Design review of the part built by this model. Coordinates are the model's own, in mm. A direction names the side the tool comes from. Coordinates: 2 decimals unless noted, no trailing zeros. Write each loop counter-clockwise with the first axis right and the second up, starting at its lowest first coordinate (ties: lowest second). Pieces come first, ordered by that corner, then holes. Notation, with made-up numbers: (-11, 43.5) - (10, 43.5) arc R33 ccw to (10, 76.5) - close; hole circle Ø3 at (61, 29.25). An arc over 180 degrees is marked (long way). Answer as a JSON object with one key per item and string values.
```python
from build123d import *

# Parameters (mm, degrees)
BOSS_EXTRUDE1_DEPTH         = 39.9
CUT_EXTRUDE1_DEPTH          = 1
CUT_EXTRUDE1_DEPTH_BACK     = 40.5
CUT_EXTRUDE2_DEPTH          = 1
CUT_EXTRUDE2_DEPTH_BACK     = 40.5
M4_TAPPED_HOLE1_D           = 3.3
M4_TAPPED_HOLE1_DEPTH       = 10.1
M4_TAPPED_HOLE1_CSINK_D     = 4.05
M4_TAPPED_HOLE1_CSINK_ANGLE = 90
M4_TAPPED_HOLE1_TIP         = 0.991420021
SKETCH6_W                   = 24.75
SKETCH6_H                   = 6.7
CUT_EXTRUDE3_DEPTH          = 2


with BuildPart() as part:
    # Sketch1 → Boss-Extrude1 (new body)
    with BuildSketch(Plane.XY):
        with BuildLine():
            Line((24.75, 0), (24.75, 14.75))
            Line((24.75, 14.75), (39.5, 14.75))
            Line((39.5, 14.75), (39.5, 39.5))
            Line((39.5, 39.5), (23.5, 39.5))
            Line((23.5, 39.5), (23.5, 20.25))
            ThreePointArc((23.5, 20.25), (22.181980515, 17.068019485), (19, 15.75))
            Line((19, 15.75), (0, 15.75))
            Line((0, 15.75), (0, 0))
            Line((0, 0), (24.75, 0))
        make_face()
    extrude(amount=BOSS_EXTRUDE1_DEPTH)

    # Sketch2 → Cut-Extrude1 (cut, two sides)
    with BuildSketch(Plane.XZ) as cut_extrude1_sk:
        with BuildLine():
            Line((10.3, 39.9), (12.3, 39.9))
            Line((12.3, 39.9), (12.3, 22.422616289))
            ThreePointArc((12.3, 22.422616289), (17.8, 16), (12.3, 9.577383711))
            Line((12.3, 9.577383711), (12.3, 2.9))
            Line((12.3, 2.9), (10.3, 2.9))
            Line((10.3, 2.9), (10.3, 9.577383711))
            ThreePointArc((10.3, 9.577383711), (4.8, 16), (10.3, 22.422616289))
            Line((10.3, 22.422616289), (10.3, 39.9))
        make_face()
    extrude(amount=CUT_EXTRUDE1_DEPTH, mode=Mode.SUBTRACT)
    extrude(cut_extrude1_sk.sketch, amount=-CUT_EXTRUDE1_DEPTH_BACK, mode=Mode.SUBTRACT)

    # Sketch3 → Cut-Extrude2 (cut, two sides)
    with BuildSketch(Plane(origin=(39.5, 0, 0), x_dir=(0, 0, -1), z_dir=(1, 0, 0))) as cut_extrude2_sk:
        with BuildLine():
            Line((-39.9, 27.2), (-30.422616289, 27.2))
            ThreePointArc((-30.422616289, 27.2), (-24, 21.7), (-17.577383711, 27.2))
            Line((-17.577383711, 27.2), (-2.55, 27.2))
            Line((-2.55, 27.2), (-2.55, 29.2))
            Line((-2.55, 29.2), (-17.577383711, 29.2))
            ThreePointArc((-17.577383711, 29.2), (-24, 34.7), (-30.422616289, 29.2))
            Line((-30.422616289, 29.2), (-39.9, 29.2))
            Line((-39.9, 29.2), (-39.9, 27.2))
        make_face()
    extrude(amount=CUT_EXTRUDE2_DEPTH, mode=Mode.SUBTRACT)
    extrude(cut_extrude2_sk.sketch, amount=-CUT_EXTRUDE2_DEPTH_BACK, mode=Mode.SUBTRACT)

    # M4 Tapped Hole1
    with Locations(Plane(origin=(0, 0, 0), x_dir=(-1, 0, 0), z_dir=(0, 0, -1))):
        with Locations((-31.75, 31.75), (-7.75, 7.75)):
            CounterSinkHole(M4_TAPPED_HOLE1_D / 2, M4_TAPPED_HOLE1_CSINK_D / 2, depth=M4_TAPPED_HOLE1_DEPTH, counter_sink_angle=M4_TAPPED_HOLE1_CSINK_ANGLE)
            with Locations((0, 0, -(M4_TAPPED_HOLE1_DEPTH + M4_TAPPED_HOLE1_TIP / 2))):  # 118° drill point
                Cone(0, M4_TAPPED_HOLE1_D / 2, M4_TAPPED_HOLE1_TIP, mode=Mode.SUBTRACT)

    # Sketch6 → Cut-Extrude3 (cut)
    with BuildSketch(Plane.XZ):
        with Locations((12.375, 36.55)):
            Rectangle(SKETCH6_W, SKETCH6_H)
    extrude(amount=-CUT_EXTRUDE3_DEPTH, mode=Mode.SUBTRACT)


solid = part.part
```
(1) Tool access review of faces 1 (the face through (31.6, 34.7, 23.9)), 2 (the face through (4.8, 7.8, 15.9)), 3 (the face through (32, 28, 2.55)), 4 (the face through (10.3, 8, 31)), 5 (the face through (23.5, 30, 15)): name each direction out of +Z, -Z, +X, -X, +Y, -Y from which nothing blocks a thin tool from reaching the whole face with its end or side.
Solved:
{"face 1": "+X, -X", "face 2": "+Y, -Y", "face 3": "+Z, +X, -X", "face 4": "+Z, +Y, -Y", "face 5": "+Z, -Z, -X, +Y"}
(2) For pin 1 (3.5 mm diameter, centred on y = 5.5, z = 7.5, fed in from +X); pin 2 (1 mm diameter, centred on x = 11.5, y = 7, fed in from +Z); pin 3 (0.6 mm diameter, centred on x = 6.5, y = 1.5, fed in from +Z), all flat-tipped, find the tip position at first contact; note any pin that passes through.
Solved:
{"pin 1": "stops at x = 24.75", "pin 2": "stops at z = 2.9", "pin 3": "stops at z = 33.2"}
(3) To check wall thickness, follow line 1 (X direction, y = 7.75, z = 5); line 2 (Y direction, x = 31.75, z = 2.75); line 3 (X direction, y = 13, z = 3). State the ranges of each line that lie inside material, in increasing order. Write a range as from..to.
Solved:
{"line 1": "x = 0..6.1, 9.4..10.3, 12.3..24.75", "line 2": "y = 14.75..27.2, 29.2..30.1, 33.4..39.5", "line 3": "x = 0..10.3, 12.3..24.75"}
(4) Take a section at B-B, the plane z = 26.5. Write out the cut boundary in (x, y), and give its area (3 significant figures).
Solved:
{"outline": "(0, 0) - (10.3, 0) - (10.3, 15.75) - (0, 15.75) - close; (12.3, 0) - (24.75, 0) - (24.75, 14.75) - (39.5, 14.75) - (39.5, 22.2) - (23.5, 22.2) - (23.5, 20.25) arc R4.5 cw to (19, 15.75) - (12.3, 15.75) - close; (23.5, 34.2) - (39.5, 34.2) - (39.5, 39.5) - (23.5, 39.5) - close", "area": "565 mm^2"}
(5) Take a section at A-A, the plane z = 5. Write out the cut boundary in (x, y).
Solved:
{"outline": "(0, 0) - (10.3, 0) - (10.3, 15.75) - (0, 15.75) - close; (12.3, 0) - (24.75, 0) - (24.75, 14.75) - (39.5, 14.75) - (39.5, 27.2) - (23.5, 27.2) - (23.5, 20.25) arc R4.5 cw to (19, 15.75) - (12.3, 15.75) - close; (23.5, 29.2) - (39.5, 29.2) - (39.5, 39.5) - (23.5, 39.5) - close; hole circle Ø3.3 at (7.75, 7.75); hole circle Ø3.3 at (31.75, 31.75)"}
(6) The part is to be moulded in two halves that separate along Y. For faces 6 (the face through (5, 15.75, 20)), 7 (the face through (32, 29.2, 10)), 8 (the face through (24.75, 7, 20)), say which applies: pulls with the +Y half, pulls with the -Y half, needs draft (parallel to the pull), parting line crosses it, or undercut.
Solved:
{"face 6": "pulls with the +Y half", "face 7": "undercut", "face 8": "needs draft"}
(7) Take a section at C-C, the plane y = 4. Write out the cut boundary in (x, z), and give its area (3 significant figures).
Solved:
{"outline": "(0, 0) - (24.75, 0) - (24.75, 39.9) - (12.3, 39.9) - (12.3, 22.42) arc R6.5 cw to (12.3, 9.58) - (12.3, 2.9) - (10.3, 2.9) - (10.3, 9.58) arc R6.5 cw to (10.3, 22.42) - (10.3, 39.9) - (0, 39.9) - close", "area": "807 mm^2"}
(8) Take a section at D-D, the plane x = 15.5. Write out the cut boundary in (y, z).
Solved:
{"outline": "(0, 0) - (15.75, 0) - (15.75, 11.04) - (0, 11.04) - close; (0, 20.96) - (15.75, 20.96) - (15.75, 39.9) - (2, 39.9) - (2, 33.2) - (0, 33.2) - close"}
